Can you work these out from the drawing? Everything is in mm from the part's minimum corner. Coordinates: 2 decimals unless noted, no trailing zeros. Order: outer loops, then holes, each group sorted by start corner. A loop starts at its lowest first (then second) coordinate and runs counter-clockwise, first axis right, second up. Notation, with made-up numbers: (-1, -7.5) -> (36, -7.5) arc R18 cw to (36, 5.5) -> close; hole circle Ø5 at (81.25, 52.5). An arc over 180 degrees is marked (long way). Put each result on its own line as item: value. Start each with the question number.
Q1. Will these pins go through, and if not, where does the flat tip stop? pin 1 (10 mm diameter, centred on x = 47.5, z = 227, fed in from -Y); pin 2 (1.9 mm diameter, centred on x = 149.5, y = 3.5, fed in from -Z); pin 3 (1.9 mm diameter, centred on y = 3.5, z = 61, fed in from +X); pin 4 (1.9 mm diameter, centred on x = 3.5, y = 2, fed in from -Z).
Q2. If we section it at A-A (y = 3): Please give me the cut outline in (x, z).
Q3. If we section it at B-B (x = 83): Please give me the cut outline in (y, z).
Q4. Please list where these lines run through material, in increasing order: line 1 along Z through (x, y) = (132, 1.75); line 2 along Z through (x, y) = (155, 5.5); line 3 along X through (y, z) = (4.75, 257.5).
Q5. If we section it at C-C (z = 58.5): Please give me the cut outline in (x, y), and give its area (3 significant figures).
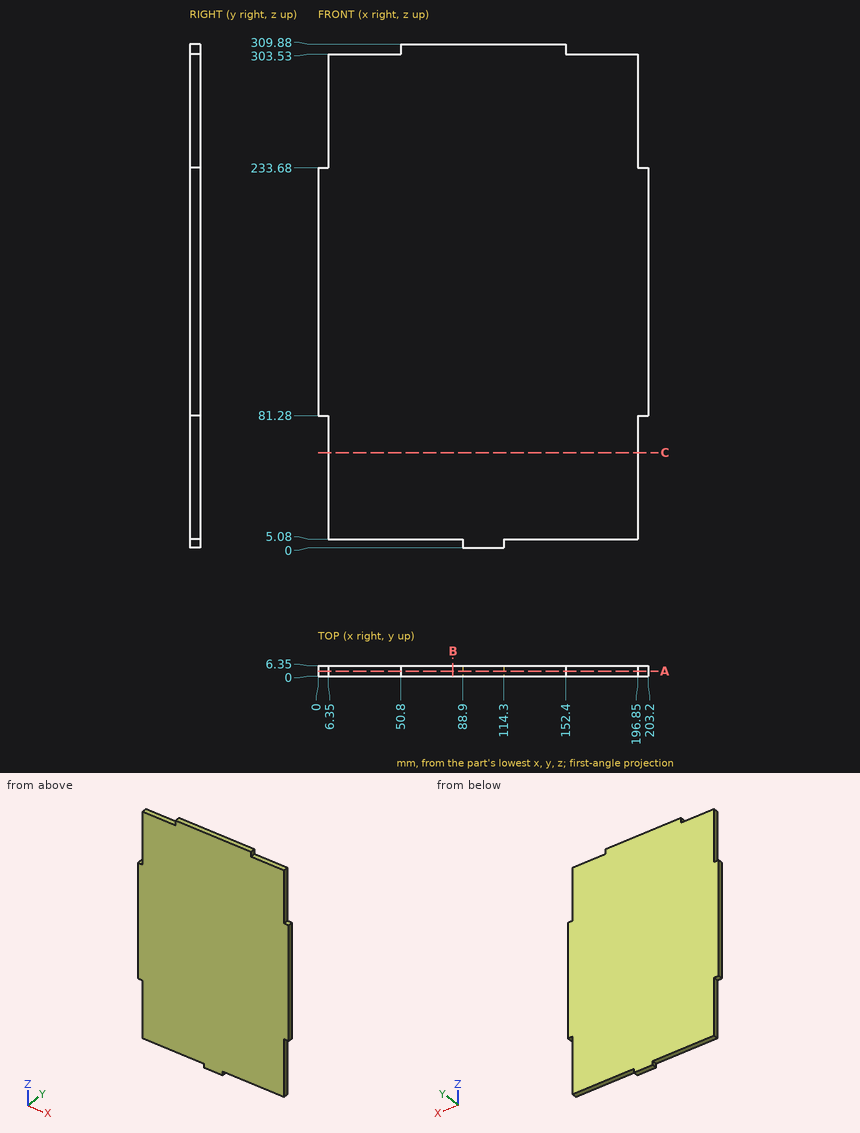
The answers:
1. pin 1: y = 0
1. pin 2: z = 5.08
1. pin 3: x = 196.85
1. pin 4: z = 81.28
2. outline: (0, 81.28) -> (6.35, 81.28) -> (6.35, 5.08) -> (88.9, 5.08) -> (88.9, 0) -> (114.3, 0) -> (114.3, 5.08) -> (196.85, 5.08) -> (196.85, 81.28) -> (203.2, 81.28) -> (203.2, 233.68) -> (196.85, 233.68) -> (196.85, 303.53) -> (152.4, 303.53) -> (152.4, 309.88) -> (50.8, 309.88) -> (50.8, 303.53) -> (6.35, 303.53) -> (6.35, 233.68) -> (0, 233.68) -> close
3. outline: (0, 5.08) -> (6.35, 5.08) -> (6.35, 309.88) -> (0, 309.88) -> close
4. line 1: 5.08 to 309.88
4. line 2: 5.08 to 303.53
4. line 3: 6.35 to 196.85
5. outline: (6.35, 0) -> (196.85, 0) -> (196.85, 6.35) -> (6.35, 6.35) -> close
5. area: 1,210 mm^2
